Design review of the part built by this model. Coordinates are the model's own, in mm. A direction names the side the tool comes from. Coordinates: 2 decimals unless noted, no trailing zeros. Order: outer loops, then holes, each group sorted by start corner. A loop starts at its lowest first (then second) coordinate and runs counter-clockwise, first axis right, second up. Notation, with made-up numbers: (23, 46.25) -> (33, 46.25) arc R30 cw to (33, 71.25) -> close; hole circle Ø2 at (31, -6). An arc over 180 degrees is marked (long way). Use a Markdown table: item, result. Add a question column.
Q1. Add section A-A (z = 0). State the section outline as (x, y) points (3 decimals).
Q2. Machinability: for faces 1 (the face through (38.12, 4.282, -0.488)), 2 (the face through (3, 12, -1)), 3 (the face through (3, 12, 1)), 4 (the face through (37, 8, -3.4)), which of the approach directions +Z, -Z, +X, -X, +Y, -Y give a long, thin tool a straight path to every point of the face, cutting with its end or side? Answer none if there is none.
Q3. The part is to be moulded in two halves that separate along X. For faces 5 (the face through (1.014, 12.868, -6.349)), 6 (the face through (37.73, 8, -3.4)), 7 (the face through (40, 8, 0)), 8 (the face through (37.37, 4.793, 0.421)), say which applies: pulls with the +X half, pulls with the -X half, needs draft (parallel to the pull), parting line crosses it, or undercut.
Q4. Add section B-B (y = 8). State the section outline as (x, z) points (3 decimals).
Q5. Add section C-C (x = 3). State the section outline as (y, z) points, then the cut area to 3 significant figures.
Q6. Wall thickness on probe 1 along X at (y, z) = (10, -3.5); probe 2 along X at (y, z) = (4.75, -0.75); probe 3 along Y at (x, z) = (36, -3): over which ranges is each line inside the solid? List them lowest first.
Q7. Add section D-D (x = 7.5). State the section outline as (y, z) points, then the cut area to 3 significant figures.
Q8. Insertion check: pin 1 (1.5 mm diameter, centred on y = 9, z = 6, fed in from +X); pin 2 (0.6 mm diameter, centred on x = 3.5, y = 12.5, fed in from -Z); pin 3 (5 mm diameter, centred on x = 21, z = -1.5, fed in from -Y); pin 4 (1 mm diameter, centred on x = 30, y = 2, fed in from +Z). Each pin has a flat end and moves straight along its axis. Give the tip position at first contact, or say it passes through.
from build123d import *

# Parameters (mm, degrees)
RIB11_REACH    = 45.818
SKETCH7_WALL_W = 92.464036326
SKETCH7_WALL_H = 2
CHAMFER1_SIZE  = 1.5
SKETCH8_W      = 0.73
SKETCH8_H      = 0.515


with BuildPart() as part:
    # Sketch1 → Revolve1 (revolve)
    with BuildSketch(Plane.XY, mode=Mode.PRIVATE) as revolve1_sk:
        Polygon((0, 0), (2, 0), (2, 4.25), (37, 4.25), (40, 4.25), (40, 8), (0, 8), align=None)
    revolve(revolve1_sk.sketch.rotate(Axis((-10.111111111, 8, 0), (1, 0, 0)), 270), axis=Axis((-10.111111111, 8, 0), (1, 0, 0)))

    # Sketch7 wall → Rib11 (add, up to next)
    with BuildSketch(Plane(origin=(3, 12.75, 0), x_dir=(0.707106781187, -0.707106781187, 0), z_dir=(0.707106781187, 0.707106781187, 0)), mode=Mode.PRIVATE) as rib11_sk1:
        Rectangle(SKETCH7_WALL_W, SKETCH7_WALL_H)
    rib11_tool1 = extrude(rib11_sk1.sketch, amount=-RIB11_REACH, mode=Mode.PRIVATE) - part.part
    add(rib11_tool1.solids().sort_by_distance((3, 12.75, 0))[0])

    # Chamfer1
    chamfer1_edges = [part.edges().sort_by_distance(p)[0] for p in [
        (40, 8, -3.75),
    ]]
    chamfer(chamfer1_edges, length=CHAMFER1_SIZE)

    # Sketch8 → Cut-Revolve1 (revolve, cut)
    with BuildSketch(Plane.XY, mode=Mode.PRIVATE) as cut_revolve1_sk:
        with Locations((37.365, 11.4925)):
            Rectangle(SKETCH8_W, SKETCH8_H)
    revolve(cut_revolve1_sk.sketch.rotate(Axis((40, 8, 0), (-1, 0, 0)), 90), axis=Axis((40, 8, 0), (-1, 0, 0)), mode=Mode.SUBTRACT)


solid = part.part
Established:
| question | item | result |
|---|---|---|
| 1 | outline | (0, 0) -> (2, 0) -> (2, 4.25) -> (37, 4.25) -> (37, 4.765) -> (37.73, 4.765) -> (37.73, 4.25) -> (38.5, 4.25) -> (40, 5.75) -> (40, 10.25) -> (38.5, 11.75) -> (37.73, 11.75) -> (37.73, 11.235) -> (37, 11.235) -> (37, 11.75) -> (4, 11.75) -> (2, 13.75) -> (2, 16) -> (0, 16) -> close |
| 2 | face 1 | +X |
| 2 | face 2 | -Z, +X, +Y |
| 2 | face 3 | +Z, +X, +Y |
| 2 | face 4 | none |
| 3 | face 5 | needs draft |
| 3 | face 6 | undercut |
| 3 | face 7 | pulls with the +X half |
| 3 | face 8 | undercut |
| 4 | outline | (0, -8) -> (2, -8) -> (2, -3.75) -> (37, -3.75) -> (37, -3.235) -> (37.73, -3.235) -> (37.73, -3.75) -> (38.5, -3.75) -> (40, -2.25) -> (40, 2.25) -> (38.5, 3.75) -> (37.73, 3.75) -> (37.73, 3.235) -> (37, 3.235) -> (37, 3.75) -> (2, 3.75) -> (2, 8) -> (0, 8) -> close |
| 5 | outline | (11.61, -1) -> (12.75, -1) -> (12.75, 1) -> (11.61, 1) arc R3.75 ccw (long way) to start |
| 5 | area | 46.3 mm^2 |
| 6 | probe 1 | 0 to 2 |
| 6 | probe 2 | 0 to 37, 37.73 to 38.91 |
| 6 | probe 3 | 5.75 to 10.25 |
| 7 | outline | circle Ø7.5 at (8, 0) |
| 7 | area | 44.2 mm^2 |
| 8 | pin 1 | x = 2 |
| 8 | pin 2 | z = -1 |
| 8 | pin 3 | y = 4.25 |
| 8 | pin 4 | through |
